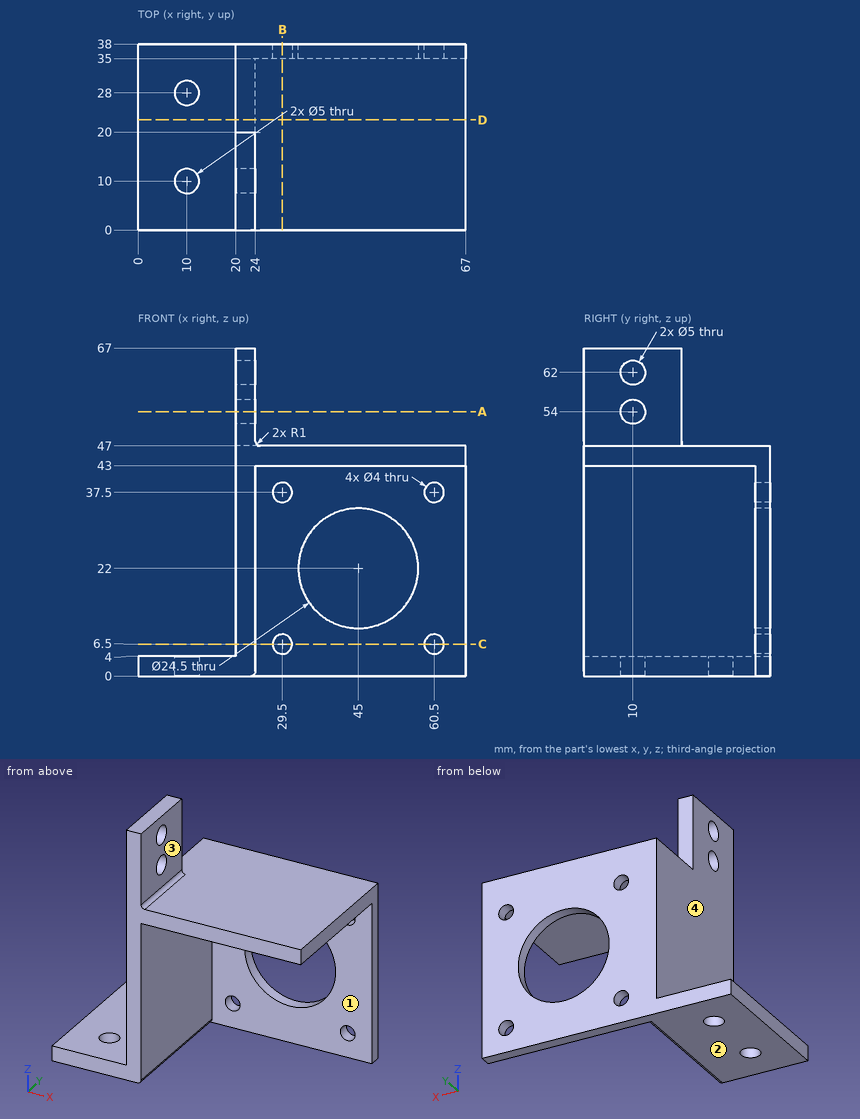
Geometry check sheet. Reference: drawing and pictorial views, mm from the part's lowest x, y, z. A direction names the side the tool comes from. Give positions to 0.01 mm unless a question says otherwise; leave off trailing zeros. Order: outer loops, then holes, each group sorted by start corner. A loop starts at its lowest first (then second) coordinate and runs counter-clockwise, first axis right, second up. Notation, with made-up numbers: M 6,-24 L 19,-24 A22 ccw 19,2 Z; hole C -14,-33 d8. An arc over 180 degrees is marked long. Answer in a Markdown table with one row per item. Add a question column.
Item 1: Tool access check on the marked faces 1, 2, 3 and 4. Record the directions out of +Z, -Z, +X, -X, +Y, -Y that give a thin tool (end or side, any length) a straight path to the whole face; none if there is none.
Item 2: Scan lines: probe 1 along Z at (x, y) = (29.5, 35.95); probe 2 along Y at (x, z) = (10, 2.1); probe 3 along X at (y, z) = (36.85, 37.5). Record each from-to range of solid material in increasing order. Write a range as from..to.
Item 3: Section check D-D, the plane y = 22.5. Enter the section's corners in (x, z).
Item 4: Gauge pin test, flat ends, axial feed: pin 1 (16 mm diameter, centred on x = 14.5, y = 17, fed in from +Z); pin 2 (8 mm diameter, centred on y = 21, z = 33.5, fed in from +X); pin 3 (5 mm diameter, centred on x = 41, y = 20, fed in from +Z); pin 4 (5.5 mm diameter, centred on x = 22.5, z = 55, fed in from +Y). Record the tip position at first contact, or that the pin passes through.
Item 5: Section check B-B, the plane x = 29.5. Enter the section's corners in (y, z).
Item 6: Section check A-A, the plane z = 54. Enter the section's corners in (x, y).
Item 7: Section check C-C, the plane z = 6.5. Enter the section's corners in (x, y), and give its area (3 significant figures).
Filled sheet:
| question | item | result |
|---|---|---|
| 1 | face 1 | -Z, +X, -Y |
| 1 | face 2 | -Z, +X, -X, +Y, -Y |
| 1 | face 3 | +Z, +X, +Y, -Y |
| 1 | face 4 | +Z, -X, +Y, -Y |
| 2 | probe 1 | z = 0..4.5, 8.5..35.5, 39.5..47 |
| 2 | probe 2 | y = 0..7.5, 12.5..25.5, 30.5..38 |
| 2 | probe 3 | x = 20..27.5, 31.5..58.5, 62.5..67 |
| 3 | outline | M 0,0 L 23,0 A1 ccw 24,1 L 24,43 L 67,43 L 67,47 L 20,47 L 20,4 L 0,4 Z |
| 4 | pin 1 | stops at z = 67 |
| 4 | pin 2 | stops at x = 24 |
| 4 | pin 3 | stops at z = 47 |
| 4 | pin 4 | stops at y = 20 |
| 5 | outline | M 0,43 L 35,43 L 35,39.5 L 38,39.5 L 38,47 L 0,47 Z; M 35,0 L 38,0 L 38,4.5 L 35,4.5 Z; M 35,8.5 L 38,8.5 L 38,35.5 L 35,35.5 Z |
| 6 | outline | M 20,0 L 24,0 L 24,7.5 L 20,7.5 Z; M 20,12.5 L 24,12.5 L 24,20 L 20,20 Z |
| 7 | outline | M 20,0 L 24,0 L 24,35 L 27.5,35 L 27.5,38 L 20,38 Z; M 31.5,35 L 58.5,35 L 58.5,38 L 31.5,38 Z; M 62.5,35 L 67,35 L 67,38 L 62.5,38 Z |
| 7 | area | 257 mm^2 |
